Can you work these out from the model? Positions are in its coordinate system, mm. Coordinates: 2 decimals unless noted, no trailing zeros. Write each loop counter-clockwise with the first axis right and the second up, starting at its lowest first coordinate (ties: lowest second). Pieces come first, ordered by that corner, then holes. Notation, with made-up numbers: (38, 37) -> (58, 37) arc R8 ccw to (58, 43) -> close; hole circle Ø3 at (-22, -2). An arc over 180 degrees is marked (long way). Answer as CSV lines item,"result". Start each with the question number.
```python
from build123d import *
from OCP.BRepFilletAPI import BRepFilletAPI_MakeChamfer

# Parameters (mm, degrees)
BOSS_EXTRU_1_DEPTH = 0.6
D_GAGEMENT_M41_D   = 4.3
CHANFREIN1_SIZE    = 0.6
CHANFREIN1_SIZE_2  = 1.039230485


with BuildPart() as part:
    # Esquisse1 → Boss.-Extru.1 (new body)
    with BuildSketch(Plane(origin=(0, 0, 0), x_dir=(1, 0, 0), z_dir=(0, 1, 0))):
        Polygon((27.5, 9.25), (35, 4.75), (35, -4.75), (27.5, -9.25), (0, -9.25), (0, 9.25), align=None)
    extrude(amount=BOSS_EXTRU_1_DEPTH)

    # Dégagement M41 (through all)
    with Locations(Plane(origin=(0, 0.6, 0), x_dir=(1, 0, 0), z_dir=(0, 1, 0))):
        with Locations((23, 0)):
            Hole(D_GAGEMENT_M41_D / 2)

    # Chanfrein1
    chanfrein1_edges_1 = [part.edges().sort_by_distance(p)[0] for p in [
        (13.75, 0.6, -9.25),
    ]]
    chanfrein1_side_1 = [part.faces().sort_by_distance(p)[0] for p in [
        (13.75, 0.588, -9.25),
    ]]
    chanfrein1_edges_2 = [part.edges().sort_by_distance(p)[0] for p in [
        (13.75, 0.6, 9.25),
    ]]
    chanfrein1_side_2 = [part.faces().sort_by_distance(p)[0] for p in [
        (13.75, 0.6, 9.238),
    ]]
    chanfrein1 = BRepFilletAPI_MakeChamfer(part.part.solid().wrapped)
    for e in chanfrein1_edges_1:
        chanfrein1.Add(CHANFREIN1_SIZE - 0.0001, CHANFREIN1_SIZE_2 - 0.0001, e.wrapped, chanfrein1_side_1[0].wrapped)
    for e in chanfrein1_edges_2:
        chanfrein1.Add(CHANFREIN1_SIZE_2 - 0.0001, CHANFREIN1_SIZE - 0.0001, e.wrapped, chanfrein1_side_2[0].wrapped)
    add(Compound.cast(chanfrein1.Shape()), mode=Mode.REPLACE)  # a hair under: the kernel refuses the full size


solid = part.part
```
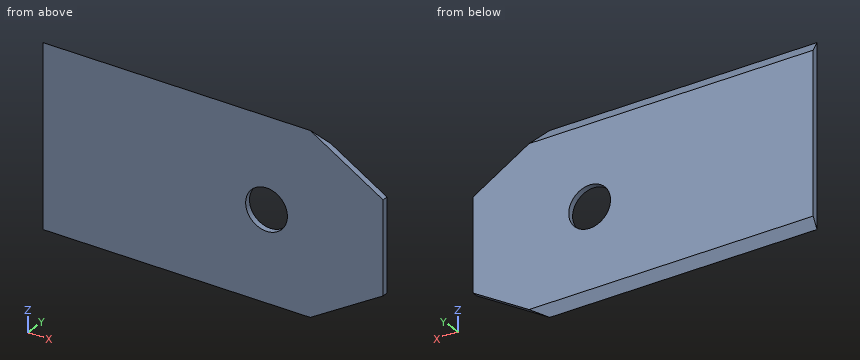
Q1. Imagine slicing it at A-A (z = 0). Write out the boundary of the cut face in (x, y), then the cut area to 3 significant figures.
Q2. Imagine slicing it at D-D (x = 30). Write out the boundary of the cut face in (y, z), then the cut area to 3 significant figures.
Q3. For pin 1 (1.5 mm diameter, centred on x = 12.5, z = 3, fed in from -Y), with a flat end and sliding along its axis, tell me the tip position at first contact or that it passes through.
Q4. I need wall thicknesses on L1, parallel to Z at x = 23, y = 0.4; L2, parallel to Z at x = 23, y = 0.2; L3, parallel to X at y = 0.25, z = -1.5. Which ranges of each line are inside material? Lowest first, please.
Q5. Imagine slicing it at C-C (y = 0.35). Write out the boundary of the cut face in (x, z).
Entries:
1,outline,"(0, 0) -> (20.85, 0) -> (20.85, 0.6) -> (0, 0.6) -> close; (25.15, 0) -> (35, 0) -> (35, 0.6) -> (25.15, 0.6) -> close"
1,area,"18.4 mm2"
2,outline,"(0, -7.75) -> (0.6, -7.75) -> (0.6, 7.75) -> (0, 7.75) -> close"
2,area,"9.30 mm2"
3,pin 1,"y = 0"
4,L1,"-8.56 to -2.15, 2.15 to 8.56"
4,L2,"-8.9 to -2.15, 2.15 to 8.9"
4,L3,"0 to 21.46, 24.54 to 35"
5,outline,"(0, -8.64) -> (28.51, -8.64) -> (35, -4.75) -> (35, 4.75) -> (28.51, 8.64) -> (0, 8.64) -> close; hole circle Ø4.3 at (23, 0)"
